Geometry check sheet. Reference: the model listing, model coordinates, mm. Coordinates: 2 decimals unless noted, no trailing zeros. Loops run counter-clockwise (first coordinate to the right, second up) from the corner with the lowest first, then second, coordinate; pieces in that order, holes last. Notation, with made-up numbers: (55, -2) - (71, -2) arc R12 cw to (71, 14) - close; hole circle Ø7 at (22.5, 11). An arc over 180 degrees is marked (long way). One line per item, written item: value.
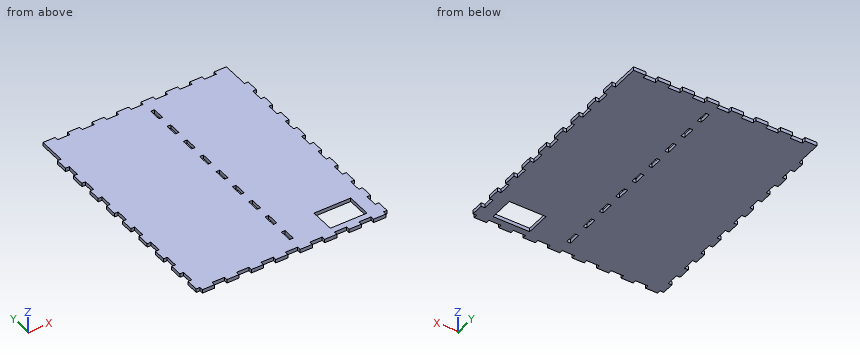
from build123d import *

# Parameters (mm, degrees)
ESQUISSE1_W                = 150
ESQUISSE1_H                = 189.15
BOSS_EXTRU_1_DEPTH         = 3
ESQUISSE2_W                = 10
ESQUISSE2_H                = 3
BOSS_EXTRU_2_DEPTH         = 3
R_P_TITION_LIN_AIRE1_COUNT = 8
R_P_TITION_LIN_AIRE1_PITCH = 20
ESQUISSE3_W                = 10
ESQUISSE3_H                = 3
BOSS_EXTRU_3_DEPTH         = 3
R_P_TITION_LIN_AIRE2_COUNT = 8
R_P_TITION_LIN_AIRE2_PITCH = 20
ESQUISSE4_W                = 3
ESQUISSE4_H                = 10
BOSS_EXTRU_4_DEPTH         = 3
R_P_TITION_LIN_AIRE3_COUNT = 9
R_P_TITION_LIN_AIRE3_PITCH = 20
ESQUISSE5_W                = 3
ESQUISSE5_H                = 10
BOSS_EXTRU_5_DEPTH         = 3
R_P_TITION_LIN_AIRE4_COUNT = 9
R_P_TITION_LIN_AIRE4_PITCH = 20
ESQUISSE6_W                = 30
ESQUISSE6_H                = 20
ENL_V_MAT_EXTRU_1_DEPTH    = 4
ESQUISSE7_W                = 3
ESQUISSE7_H                = 10
ENL_V_MAT_EXTRU_2_DEPTH    = 4
R_P_TITION_LIN_AIRE5_COUNT = 9
R_P_TITION_LIN_AIRE5_PITCH = 20


with BuildPart() as part:
    # Esquisse1 → Boss.-Extru.1 (new body)
    with BuildSketch(Plane.XY):
        with Locations((75, -94.575)):
            Rectangle(ESQUISSE1_W, ESQUISSE1_H)
    extrude(amount=BOSS_EXTRU_1_DEPTH)

    # Esquisse2 → Boss.-Extru.2 (add)
    with BuildSketch(Plane(origin=(0, 0, 0), x_dir=(1, 0, 0), z_dir=(0, 1, 0))):
        with Locations((5, -1.5)):
            Rectangle(ESQUISSE2_W, ESQUISSE2_H)
    boss_extru_2 = extrude(amount=BOSS_EXTRU_2_DEPTH)

    # Répétition linéaire1: Boss.-Extru.2 ×8
    with Locations(*[(i * R_P_TITION_LIN_AIRE1_PITCH, 0, 0) for i in range(1, R_P_TITION_LIN_AIRE1_COUNT)]):
        add(boss_extru_2)

    # Esquisse3 → Boss.-Extru.3 (add)
    with BuildSketch(Plane.XZ.offset(189.15)):
        with Locations((5, 1.5)):
            Rectangle(ESQUISSE3_W, ESQUISSE3_H)
    boss_extru_3 = extrude(amount=BOSS_EXTRU_3_DEPTH)

    # Répétition linéaire2: Boss.-Extru.3 ×8
    with Locations(*[(i * R_P_TITION_LIN_AIRE2_PITCH, 0, 0) for i in range(1, R_P_TITION_LIN_AIRE2_COUNT)]):
        add(boss_extru_3)

    # Esquisse4 → Boss.-Extru.4 (add)
    with BuildSketch(Plane.ZY):
        with Locations((1.5, -184.15)):
            Rectangle(ESQUISSE4_W, ESQUISSE4_H)
    boss_extru_4 = extrude(amount=BOSS_EXTRU_4_DEPTH)

    # Répétition linéaire3: Boss.-Extru.4 ×9
    with Locations(*[(0, i * R_P_TITION_LIN_AIRE3_PITCH, 0) for i in range(1, R_P_TITION_LIN_AIRE3_COUNT)]):
        add(boss_extru_4)

    # Esquisse5 → Boss.-Extru.5 (add)
    with BuildSketch(Plane(origin=(150, 0, 0), x_dir=(0, 0, -1), z_dir=(1, 0, 0))):
        with Locations((-1.5, -184.15)):
            Rectangle(ESQUISSE5_W, ESQUISSE5_H)
    boss_extru_5 = extrude(amount=BOSS_EXTRU_5_DEPTH)

    # Répétition linéaire4: Boss.-Extru.5 ×9
    with Locations(*[(0, i * R_P_TITION_LIN_AIRE4_PITCH, 0) for i in range(1, R_P_TITION_LIN_AIRE4_COUNT)]):
        add(boss_extru_5)

    # Esquisse6 → Enlèv. mat.-Extru.1 (cut, through all)
    with BuildSketch(Plane(origin=(0, 0, 0), x_dir=(-1, 0, 0), z_dir=(0, 0, -1))):
        with Locations((-125, -174.15)):
            Rectangle(ESQUISSE6_W, ESQUISSE6_H)
    extrude(amount=-ENL_V_MAT_EXTRU_1_DEPTH, mode=Mode.SUBTRACT)

    # Esquisse7 → Enlèv. mat.-Extru.2 (cut, through all)
    with BuildSketch(Plane(origin=(0, 0, 0), x_dir=(-1, 0, 0), z_dir=(0, 0, -1))):
        with Locations((-81.5, -14.15)):
            Rectangle(ESQUISSE7_W, ESQUISSE7_H)
    enl_v_mat_extru_2 = extrude(amount=-ENL_V_MAT_EXTRU_2_DEPTH, mode=Mode.SUBTRACT)

    # Répétition linéaire5: Enlèv. mat.-Extru.2 ×9
    with Locations(*[(0, -i * R_P_TITION_LIN_AIRE5_PITCH, 0) for i in range(1, R_P_TITION_LIN_AIRE5_COUNT)]):
        add(enl_v_mat_extru_2, mode=Mode.SUBTRACT)


solid = part.part
(1) Cross-section at D-D on z = 2.2. State how many separate pieces and enclosed holes the cut face has, and give its area (3 significant figures).
Reply:
separate pieces: 1
enclosed holes: 10
area: 28,500 mm2
(2) Cross-section at C-C on x = 77.5. Record the cut outline in (y, z), and give its area (3 significant figures).
Reply:
outline: (-189.15, 0) - (0, 0) - (0, 3) - (-189.15, 3) - close
area: 567 mm2
(3) Cross-section at A-A on y = -132.5. Record the cut outline in (x, z).
Reply:
outline: (0, 0) - (80, 0) - (80, 3) - (0, 3) - close; (83, 0) - (150, 0) - (150, 3) - (83, 3) - close
(4) Cross-section at B-B on x = 113. Record the cut outline in (y, z), and give its area (3 significant figures).
Reply:
outline: (-189.15, 0) - (-184.15, 0) - (-184.15, 3) - (-189.15, 3) - close; (-164.15, 0) - (0, 0) - (0, 3) - (-164.15, 3) - close
area: 507 mm2
(5) Go/stop test with flat-tipped pins: pin 1 Ø0.9 at (y, z) = (-35, 1.5) entering from -X; pin 2 Ø0.9 at (y, z) = (1.5, 1.5) entering from +X; pin 3 Ø10 at (x, y) = (130, -158) entering from -Z; pin 4 Ø0.9 at (x, z) = (-1.5, 2) entering from -Y. Record where each tip stops, or that it passes through.
Reply:
pin 1: x = 0
pin 2: x = 150
pin 3: z = 0
pin 4: y = -189.15
(6) Material ranges on probe 1 along X at (y, z) = (-177, 0.2); probe 2 along X at (y, z) = (-78, 2.1); probe 3 along X at (y, z) = (-179.5, 1.55), recorded low to high. Write a range as from..to.
Reply:
probe 1: 0..80, 83..110, 140..150
probe 2: 0..80, 83..150
probe 3: -3..110, 140..153
